Autodesk Inventor part; units mm, degrees
ref_plane "YZ Plane" through (0, 0, 0) normal (1, 0, 0) x (0, 1, 0)
ref_plane "XZ Plane" through (0, 0, 0) normal (0, 1, 0) x (-1, 0, 0)
ref_plane "XY Plane" through (0, 0, 0) normal (0, 0, 1) x (1, 0, 0)
sketch "Sketch1" plane through (0, 0, 0) normal (0, 1, 0) x (-1, 0, 0)
  circle A0 centre (0, 0) radius 12 construction
  line L0 (0, 0) -> (0, -50) construction
  line L1 (20, -50) -> (34, -50) construction
  line L2 (34, -50) -> (34, -16) construction
  line L3 (34, -16) -> (20, -16) construction
  line L4 (20, -16) -> (20, -50) construction
  line L5 (21, -42) -> (34, -42)
  circle A1 centre (0, 0) radius 6 construction
  line L6 (16, -14) -> (28.0909, 0.6564)
  line L7 (39, -22.4853) -> (39, -37)
  line L8 (16, -37) -> (16, -14)
  arc A2 (16, -14) -> (0, -6) centre (0, -26) ccw construction
  arc A3 (39, -22.4853) -> (28.0909, 0.6564) centre (9, -22.4853) ccw
  arc A4 (34, -42) -> (39, -37) centre (34, -37) ccw
  arc A5 (16, -37) -> (21, -42) centre (21, -37) ccw
  point P0 (16, -42)
  point P1 (39, -42)
  dimension "d26" = 12
  dimension "d0" = 50
  dimension "d1" = 24
  dimension "d16" = 16
  dimension "d17" = 34
  dimension "d18" = 23
  dimension "d19" = 26
  dimension "d21" = 5
  dimension "d23" = 20
  dimension "d25" = 16
  dimension "d27" = 30
  dimension "d28" = 19
  dimension "d30" = 5
  dimension "d31" = 5
  dimension "d32" = 20
extrude "Extrusion1" add sketch "Sketch1" along normal blind 2
properties part number "flange_small"
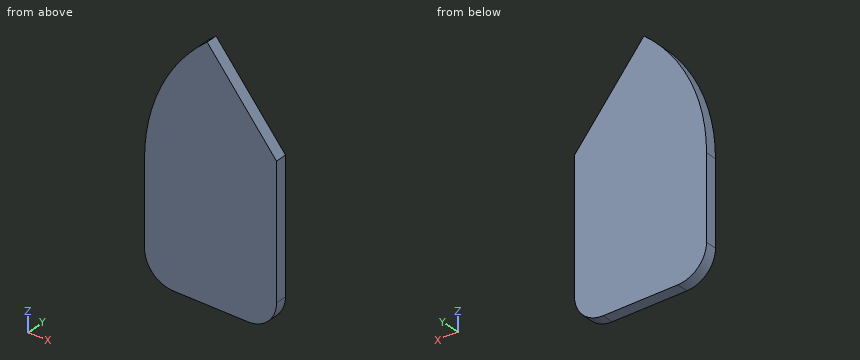
The listing builds one solid part. Answer for the finished solid, in the listing's coordinates (mm). Coordinates: 2 decimals unless noted, no trailing zeros. Write each loop counter-clockwise with the first axis right and the second up, starting at its lowest first coordinate (ties: lowest second). Pieces come first, ordered by that corner, then holes. Notation, with made-up numbers: (56.5, 25.25) - (62.5, 25.25) arc R26 ccw to (62.5, 51.25) - close; hole circle Ø7 at (12, 88.5). An arc over 180 degrees is marked (long way). Return JSON: item names as keys, results as strings.
1. This flat-tipped pin is pushed along its axis until it touches: pin 1 Ø1.5 at (x, z) = (-36.5, -25) entering from -Y. Where does it stop, or does it pass through?
Final values:
{"pin 1": "y = 0"}
2. The part is cut by section A-A on y = 0.4. Determine the outline of the cut face in (x, z), then the cut area to 3 significant figures.
Final values:
{"outline": "(-39, -37) arc R5 ccw to (-34, -42) - (-21, -42) arc R5 ccw to (-16, -37) - (-16, -14) - (-28.09, 0.66) arc R30 ccw to (-39, -22.49) - close", "area": "805 mm^2"}
3. The part is cut by section C-C on z = -2.5. Determine the outline of the cut face in (x, y).
Final values:
{"outline": "(-31.37, 0) - (-25.49, 0) - (-25.49, 2) - (-31.37, 2) - close"}
4. Consider line 1 along X through (y, z) = (1.3, -22); line 2 along X through (y, z) = (1.5, -4.5); line 3 along Z through (x, y) = (-28.75, 0.6). Determine where each line is inside the solid, lowest interval first.
Final values:
{"line 1": "-39 to -16", "line 2": "-33.01 to -23.84", "line 3": "-42 to 0.1"}
5. The part is cut by section B-B on x = -27.25. Determine the outline of the cut face in (y, z), then the cut area to 3 significant figures.
Final values:
{"outline": "(0, -42) - (2, -42) - (2, -0.36) - (0, -0.36) - close", "area": "83.3 mm^2"}
